from build123d import *

# Parameters (mm, degrees)
SKETCH1_R           = 0.2
BOSS_EXTRUDE1_DEPTH = 0.8


with BuildPart() as part:
    # Sketch1 → Boss-Extrude1 (new body)
    with BuildSketch(Plane(origin=(0, 0, 0), x_dir=(1, 0, 0), z_dir=(0, 1, 0))):
        with BuildLine():
            ThreePointArc((-2.383636789, 23.134738828), (-2.370326041, 23.784413457), (-2.565996752, 24.404064385))
            ThreePointArc((-2.565996752, 24.404064385), (-0.19892847, 34.515692649), (-0.514652369, 44.895883246))
            ThreePointArc((-0.514652369, 44.895883246), (-1.342299158, 46.382879838), (-2.929984682, 46.995589192))
            ThreePointArc((-2.929984682, 46.995589192), (-5.811012003, 46.848007958), (-8.640837363, 46.287484025))
            ThreePointArc((-8.640837363, 46.287484025), (-7.900405237, 35.032644788), (-6.316363211, 23.865261172))
            ThreePointArc((-6.316363211, 23.865261172), (-6.329673959, 23.215586543), (-6.134003248, 22.595935615))
            ThreePointArc((-6.134003248, 22.595935615), (-8.50107153, 12.484307351), (-8.185347631, 2.104116754))
            ThreePointArc((-8.185347631, 2.104116754), (-7.357700842, 0.617120162), (-5.770015318, 0.004410808))
            ThreePointArc((-5.770015318, 0.004410808), (-2.888987997, 0.151992042), (-0.059162637, 0.712515975))
            ThreePointArc((-0.059162637, 0.712515975), (-0.799594763, 11.967355212), (-2.383636789, 23.134738828))
        make_face()
        with Locations((-4.35, 23.5)):
            Circle(SKETCH1_R, mode=Mode.SUBTRACT)
    extrude(amount=BOSS_EXTRUDE1_DEPTH)


solid = part.part
The listing builds one solid part. Answer for the finished solid, in the listing's coordinates (mm). A direction names the side the tool comes from. Coordinates: 2 decimals unless noted, no trailing zeros. Write each loop counter-clockwise with the first axis right and the second up, starting at its lowest first coordinate (ties: lowest second). Pieces come first, ordered by that corner, then holes. Notation, with made-up numbers: (6.5, -37) - (46.5, -37) arc R16 cw to (46.5, -18) - close; hole circle Ø5 at (50.5, -30.75). An arc over 180 degrees is marked (long way). Answer as CSV lines item,"result".
1. Determine the mould class of faces 4 (the cylindrical face through (-7.376, 0.394, -0.633)), 5 (the flat face through (-4, 0.8, -24)), 6 (the cylindrical face through (-8.486, 0.394, -12.629)), 7 (the cylindrical face through (-1.324, 0.394, -46.367)) for opening direction Z: +Z half, -Z half, draft (parallel to the pull), parting line (faces both ways), or undercut.
Computed values:
face 4,"+Z half"
face 5,"draft"
face 6,"undercut"
face 7,"-Z half"
2. Find section D-D (z = -30.5). Give the vertices of the cut face in (x, y).
Computed values:
outline,"(-7.36, 0) - (-0.81, 0) - (-0.81, 0.8) - (-7.36, 0.8) - close"
3. A tool of negligible diameter and unlimited length cuts with its end or side. For faces 1 (the cylindrical face through (-0.783, 0.394, -11.81)), 2 (the flat face through (-4, 0, -24)), 3 (the cylindrical face through (-7.917, 0.394, -35.19)), from which of +Z, -Z, +X, -X, +Y, -Y can it reach the whole face along a straight path? Write none if from no direction.
Computed values:
face 1,"+X, +Y, -Y"
face 2,"+Z, -Z, +X, -X, -Y"
face 3,"-X, +Y, -Y"
4. Find section C-C (z = -12). Give the vertices of the cut face in (x, y), plus the area to 3 significant figures.
Computed values:
outline,"(-8.55, 0) - (-0.8, 0) - (-0.8, 0.8) - (-8.55, 0.8) - close"
area,"6.19 mm²"
5. Find section A-A (y = 0.65). Give the vertices of the cut face in (x, z), plus the area to 3 significant figures.
Computed values:
outline,"(-8.64, -46.29) arc R20 ccw to (-2.93, -47) arc R2.5 ccw to (-0.51, -44.9) arc R40 ccw to (-2.57, -24.4) arc R2 ccw to (-2.38, -23.13) arc R150 ccw to (-0.06, -0.71) arc R20 ccw to (-5.77, 0) arc R2.5 ccw to (-8.19, -2.1) arc R40 ccw to (-6.13, -22.6) arc R2 ccw to (-6.32, -23.87) arc R150 ccw to start; hole circle Ø0.4 at (-4.35, -23.5)"
area,"327 mm²"
6. Find section B-B (x = -7.5). Give the vertices of the cut face in (y, z), plus the area to 3 significant figures.
Computed values:
outline,"(0, -46.56) - (0.8, -46.56) - (0.8, -31.56) - (0, -31.56) - close; (0, -18.22) - (0.8, -18.22) - (0.8, -0.75) - (0, -0.75) - close"
area,"26.0 mm²"
7. Straight lines are drawn through the part: line 1 (X direction, y = 0.3, z = -23.5); line 2 (Z direction, x = -4.35, y = 0.45); line 3 (Z direction, x = -2.75, y = 0.7). For each, find the intervals that lie inside material, in ascending order. Write a range as [from, to].
Computed values:
line 1,"x = [-6.35, -4.55], [-4.15, -2.35]"
line 2,"z = [-46.97, -23.7], [-23.3, -0.03]"
line 3,"z = [-46.99, -0.17]"
